The figure shows three views and two pictorial views of one solid part (mm, origin at its lowest corner). Answer the questions. Coordinates: 2 decimals unless noted, no trailing zeros. Order: outer loops, then holes, each group sorted by start corner. A loop starts at its lowest first (then second) coordinate and runs counter-clockwise, first axis right, second up. Notation, with made-up numbers: M 83,13 L 128,13 A6 cw 128,17 Z; hole C 23.25,-23 d5. An arc over 180 degrees is marked long. Use a Markdown table: item, result.
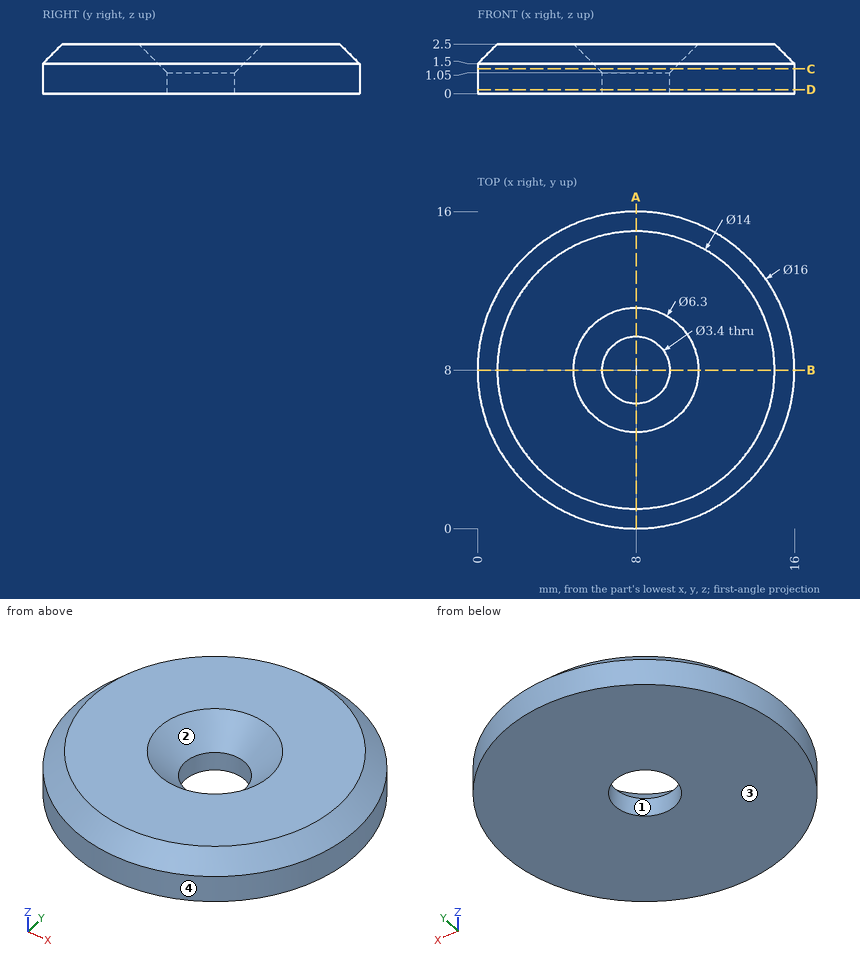
1. Section C-C on z = 1.25 is taken. Determine the outline of the cut face in (x, y), then the cut area to 3 significant figures.
Answers below:
| item | result |
|---|---|
| outline | C 8,8 d16; hole C 8,8 d3.8 |
| area | 190 mm² |
2. Section D-D on z = 0.2 is taken. Determine the outline of the cut face in (x, y).
Answers below:
| item | result |
|---|---|
| outline | C 8,8 d16; hole C 8,8 d3.4 |
3. Find the intervals of material crossed by probe 1 along Y at (x, z) = (8, 0.3); probe 2 along Y at (x, z) = (9.75, 1.35); probe 3 along X at (y, z) = (8.5, 0.25), in increasing order.
Answers below:
| item | result |
|---|---|
| probe 1 | 0 to 6.3, 9.7 to 16 |
| probe 2 | 0.19 to 7.03, 8.97 to 15.81 |
| probe 3 | 0.02 to 6.38, 9.62 to 15.98 |
4. Flat-ended cylindrical pins translate along their axes: P1, Ø4, axis at x = 8, y = 8, coming from the +Z side; P2, Ø1, axis at x = 10.5, z = 0.5, coming from the +Y side. Find the tip coordinate at first contact, or state that the pin passes through.
Answers below:
| item | result |
|---|---|
| P1 | z = 1.35 |
| P2 | y = 15.75 |
5. Section A-A on x = 8 is taken. Determine the outline of the cut face in (y, z).
Answers below:
| item | result |
|---|---|
| outline | M 0,0 L 6.3,0 L 6.3,1.05 L 4.85,2.5 L 1,2.5 L 0,1.5 Z; M 9.7,0 L 16,0 L 16,1.5 L 15,2.5 L 11.15,2.5 L 9.7,1.05 Z |
6. For a pull along X with two mould halves and no side action, classify the marked faces 1, 2, 3 and 4 as +X half, -X half, draft (parallel to the pull), parting line (faces both ways), or undercut.
Answers below:
| item | result |
|---|---|
| face 1 | undercut |
| face 2 | undercut |
| face 3 | draft |
| face 4 | parting line |
